Geometry: final body of the model. Coordinates: model frame, mm. A direction names the side the tool comes from. Round coordinates to 2 decimals unless told otherwise and drop trailing zeros. Order: outer loops, then holes, each group sorted by start corner. A loop starts at its lowest first (then second) coordinate and runs counter-clockwise, first axis right, second up. Notation, with made-up numbers: (67.5, 14.25) -> (106.5, 14.25) arc R15 cw to (106.5, 28.25) -> close; hole circle Ø9 at (19, 78.25). An arc over 180 degrees is marked (long way). Put each result on its own line as item: value.
Autodesk Inventor part; units mm, degrees
ref_plane "YZ Plane" through (0, 0, 0) normal (1, 0, 0) x (0, 1, 0)
ref_plane "XZ Plane" through (0, 0, 0) normal (0, 1, 0) x (-1, 0, 0)
ref_plane "XY Plane" through (0, 0, 0) normal (0, 0, 1) x (1, 0, 0)
sketch "Sketch1" plane through (0, 0, 0) normal (0, 0, 1) x (1, 0, 0)
  line L0 (0, 0) -> (704.681, 0) construction
  line L1 (704.681, 0) -> (704.681, 101.6) construction
  line L2 (704.681, 101.6) -> (0, 101.6) construction
  circle A0 centre (304.8, 38.1) radius 38.1 construction
  circle A1 centre (212.725, 197.5786) radius 38.1 construction
  circle A2 centre (274.2046, 266.7) radius 38.1 construction
  circle A3 centre (499.5893, 180.5177) radius 203.2 construction
  line L3 (78.3329, 304.8) -> (550.894, 304.8) construction
  circle A4 centre (247.764, 111.4893) radius 57.15 construction
  circle A5 centre (258.7625, 117.8393) radius 53.975 construction
  line L4 (212.725, 197.5786) -> (304.8, 38.1) construction
  line L5 (258.7625, 117.8393) -> (247.764, 111.4893) construction
  line L6 (274.2046, 266.7) -> (212.725, 197.5786) construction
  dimension "d0" = 101.6
  dimension "d2" = 76.2
  dimension "d3" = 76.2
  dimension "d4" = 76.2
  dimension "d8" = 406.4
  dimension "d9" = 304.8
  dimension "d11" = 304.8
  dimension "d13" = 114.3
  dimension "d14" = 107.95
  dimension "d15" = 12.7
  dimension "d16" = 92.5068
  dimension "d17" = 60
sketch "Sketch4" plane through (0, 0, 0) normal (0, 0, 1) x (1, 0, 0)
  circle A0 centre (274.2046, 266.7) radius 38.1 construction
  circle A1 centre (212.725, 197.5786) radius 38.1 construction
  circle A2 centre (247.764, 111.4893) radius 57.15 construction
  circle A3 centre (304.8, 38.1) radius 38.1 construction
  circle A4 centre (274.2046, 266.7) radius 14.2875
  circle A5 centre (212.725, 197.5786) radius 14.2875
  circle A6 centre (304.8, 38.1) radius 14.2875
  circle A7 centre (145.2547, 121.0056) radius 39.6875 construction
  circle A8 centre (165.2583, 44.1925) radius 39.6875 construction
  circle A9 centre (145.2547, 121.0056) radius 14.2875
  circle A10 centre (165.2583, 44.1925) radius 14.2875
  line L0 (304.8, 38.1) -> (165.2583, 44.1925) construction
  line L1 (145.2547, 121.0056) -> (212.725, 197.5786) construction
  circle A11 centre (165.2583, 44.1925) radius 23.876 construction
  circle A12 centre (145.2547, 121.0056) radius 23.876 construction
  line L2 (128.9029, 138.4033) -> (202.94, 207.9895) construction
  line L3 (164.5725, 106.974) -> (224.2849, 189.182) construction
  line L4 (165.8568, 20.324) -> (305.1581, 23.817) construction
  line L5 (306.4016, 52.2974) -> (167.9348, 67.918) construction
  circle A13 centre (120.0426, 37.9792) radius 5.9531 construction
  circle A14 centre (120.0426, 37.9792) radius 25.4 construction
  circle A15 centre (117.2754, 69.6084) radius 6.35 construction
  circle A16 centre (122.8098, 6.35) radius 6.35 construction
  line L6 (117.2754, 69.6084) -> (122.8098, 6.35) construction
  line L7 (0, 0) -> (304.8, 0) construction
  line L8 (69.2426, 0) -> (94.6426, 0) construction
  line L9 (94.6426, 0) -> (94.6426, 152.4) construction
  line L10 (94.6426, 152.4) -> (69.2426, 152.4)
  line L11 (69.2426, 152.4) -> (69.2426, 0)
  line L12 (81.9426, 127) -> (81.9426, 25.4) construction
  line L13 (283.8015, 39.0168) -> (325.7985, 37.1832) construction
  line L14 (260.2358, 250.9949) -> (288.1734, 282.4051) construction
  line L15 (145.2547, 99.9871) -> (145.2547, 142.0241) construction
  line L16 (165.2583, 23.174) -> (165.2583, 65.211) construction
  line L17 (226.6204, 213.3487) -> (198.8296, 181.8085) construction
  circle A17 centre (304.8, 38.1) radius 26.9875 construction
  circle A18 centre (325.7985, 37.1832) radius 12.7 construction
  circle A19 centre (288.1734, 282.4051) radius 12.7 construction
  line L18 (274.2046, 266.7) -> (212.725, 197.5786) construction
  circle A20 centre (274.2046, 266.7) radius 26.9875 construction
  circle A21 centre (212.725, 197.5786) radius 26.9875 construction
  arc A22 (94.6426, 152.4) -> (188.7085, 209.8884) centre (94.6426, 258.1022) ccw
  line L19 (254.0394, 284.6358) -> (192.5598, 215.5143)
  arc A23 (280.9291, 292.8363) -> (254.0394, 284.6358) centre (274.2046, 266.7) ccw
  arc A24 (299.3783, 276.4268) -> (280.9291, 292.8363) centre (288.1734, 282.4051) ccw
  line L20 (205.2733, 149.7079) -> (294.2696, 248.6523)
  arc A25 (205.2733, 149.7079) -> (260.3346, 55.7389) centre (247.764, 111.4893) ccw
  line L21 (260.3346, 55.7389) -> (298.8639, 64.4266)
  arc A26 (294.2696, 248.6523) -> (299.3783, 276.4268) centre (274.2046, 266.7) ccw
  arc A27 (192.5598, 215.5143) -> (188.7085, 209.8884) centre (212.725, 197.5786) ccw
  arc A28 (329.3139, 49.387) -> (298.8639, 64.4266) centre (304.8, 38.1) ccw
  arc A29 (328.2369, 24.7195) -> (329.3139, 49.387) centre (325.7985, 37.1832) ccw
  line L22 (306.4392, 11.1623) -> (123.1955, 0.0117)
  line L23 (69.2426, 0) -> (122.8098, 0)
  arc A30 (122.8098, 0) -> (123.1955, 0.0117) centre (122.8098, 6.35) ccw
  arc A31 (306.4392, 11.1623) -> (328.2369, 24.7195) centre (304.8, 38.1) ccw
  circle A32 centre (120.0426, 37.9792) radius 9.525
  circle A33 centre (120.0426, 37.9792) radius 17.4625 construction
  circle A34 centre (260.3923, 40.0389) radius 6.35 construction
  point P0 (81.9426, 76.2)
  point P1 (94.6426, 76.2)
  point P2 (81.9426, 152.4)
  point P3 (243.4648, 232.1393)
  point P4 (118.5207, 55.3752)
  point P5 (178.9898, 159.2921)
  point P6 (104.2162, 45.3592)
  point P7 (105.7382, 27.9631)
  point P8 (121.5646, 20.5831)
  point P9 (135.869, 30.5992)
  point P10 (134.3471, 47.9953)
  dimension "d81" = 34.925
  dimension "d63" = 28.575
  dimension "d64" = 79.375
  dimension "d65" = 47.752
  dimension "d66" = 139.6746
  dimension "d67" = 102.0572
  dimension "d68" = 11.9062
  dimension "d69" = 50.8
  dimension "d70" = 12.7
  dimension "d71" = 2.5
  dimension "d72" = 85
  dimension "d73" = 25.4
  dimension "d74" = 152.4
  dimension "d75" = 101.6
  dimension "d76" = 42.037
  dimension "d77" = 12.7
  dimension "d79" = 25.4
  dimension "d80" = 19.05
  dimension "d92" = 12.7
  dimension "d95" = 360
extrude "Extrusion2" add sketch "Sketch4" along normal blind 6.35
hole "Hole2" at (117.2754, 69.6084, 0) at (122.8098, 6.35, 0) at (81.9426, 127, 0) at (81.9426, 76.2, 0) at (81.9426, 25.4, 0) at (283.8015, 39.0168, 0) at (325.7985, 37.1832, 0) at (260.2358, 250.9949, 0) at (288.1734, 282.4051, 0) at (145.2547, 142.0241, 0) at (145.2547, 99.9871, 0) at (165.2583, 65.211, 0) at (165.2583, 23.174, 0) at (198.8296, 181.8085, 0) at (226.6204, 213.3487, 0) at (243.4648, 232.1393, 0) at (118.5207, 55.3752, 0) at (260.3923, 40.0389, 0) at (178.9898, 159.2921, 0) at (134.3471, 47.9953, 0) at (135.869, 30.5992, 0) at (121.5646, 20.5831, 0) at (105.7382, 27.9631, 0) at (104.2162, 45.3592, 0) direction (0, 0, 1) diameter 5.1054 end through all
fillet "Fillet2" radius 25.4 4 edges at (299.3783, 276.4268, 3.175) (280.9291, 292.8363, 3.175) (329.3139, 49.387, 3.175) (328.2369, 24.7195, 3.175)
properties part number "GP8-001" material "Polycarbonate, Smoke"
1. Cut plane B-B on x = 219.5. Return loops of the section in (y, z), and give its area (3 significant figures).
Ans:
outline: (5.87, 0) -> (61.82, 0) -> (61.82, 6.35) -> (5.87, 6.35) -> close; (165.52, 0) -> (185, 0) -> (185, 6.35) -> (165.52, 6.35) -> close; (210.16, 0) -> (245.8, 0) -> (245.8, 6.35) -> (210.16, 6.35) -> close
area: 705 mm²
2. Contact query for flat-ended pins moving along their axis: P1, Ø6, axis at x = 165.26, y = 65.21, coming from the -Z side; P2, Ø4, axis at x = 260.39, y = 40.04, coming from the -Z side; P3, Ø1.5, axis at x = 214.5, z = 4.5, coming from the +Y side; P4, Ø1, axis at x = 292.5, z = 5.5, coming from the -Y side. Output: stop coordinate, or through.
Ans:
P1: z = 0
P2: through
P3: y = 241.02
P4: y = 10.28
3. Set-up query: faces 1 (the face through (223.73, 250.56, 3.13)), 2 (the face through (249.15, 198.49, 3.13)), 3 (the face through (279.33, 60.02, 3.13)). Return all of +Z, -Z, +X, -X, +Y, -Y with unobstructed straight access to the full face (end or side cutting, diameter ignored); none if empty.
Ans:
face 1: +Z, -Z, -X, +Y
face 2: +Z, -Z, +X
face 3: +Z, -Z
4. Cut plane A-A on y = 117.5. Return loops of the section in (x, z), and give its area (3 significant figures).
Ans:
outline: (69.24, 0) -> (131.4, 0) -> (131.4, 6.35) -> (69.24, 6.35) -> close; (159.11, 0) -> (190.93, 0) -> (190.93, 6.35) -> (159.11, 6.35) -> close
area: 597 mm²
5. Material intervals for probe 1 along X at (y, z) = (198, 1.5); probe 2 along Y at (x, z) = (244.5, 5); probe 3 along X at (y, z) = (22, 5.25), sorted ascending.
Ans:
probe 1: 181.59 to 198.44, 227.01 to 248.71
probe 2: 7.39 to 54.43, 193.32 to 229.81, 234.47 to 273.91
probe 3: 69.24 to 119.44, 123.69 to 162.99, 167.53 to 326.64
6. Cut plane C-C on z = 2.5. State how many separate pieces and enclosed holes the cut face has, and give its area (3 significant figures).
Ans:
separate pieces: 1
enclosed holes: 30
area: 31,700 mm²
7. Cut plane D-D on y = 266.7. Return loops of the section in (x, z).
Ans:
outline: (238.09, 0) -> (259.92, 0) -> (259.92, 6.35) -> (238.09, 6.35) -> close; (288.49, 0) -> (301.19, 0) -> (301.19, 6.35) -> (288.49, 6.35) -> close
8. Draft query along Y for faces 4 (the face through (216.1, 5.665, 3.131)), 5 (the face through (134.724, 111.349, 3.131)), 6 (the face through (82, 152.4, 3)), 7 (the face through (220.406, 185.531, 3.131)). Return one class per face: +Y half, -Y half, draft (parallel to the pull), parting line (faces both ways), or undercut.
Ans:
face 4: -Y half
face 5: undercut
face 6: +Y half
face 7: undercut
